Read the model definition and answer for the solid it produces. Units are mm, in the model's axes. Coordinates: 2 decimals unless noted, no trailing zeros. Write each loop counter-clockwise with the first axis right and the second up, starting at its lowest first coordinate (ties: lowest second). Pieces come first, ordered by that corner, then holes. Notation, with made-up numbers: (56, -22) -> (79, -22) arc R19 ccw to (79, -16) -> close; hole circle Ø6 at (-4.75, 5.25). An arc over 180 degrees is marked (long way). Use CSV: the item, a comma, the result in double quotes.
from build123d import *

# Parameters (mm, degrees)
F0_R     = 1.6
F1_DEPTH = 3.175


with BuildPart() as f1:
    # F0 (on Top) → F1 (new body)
    with BuildSketch(Plane.XY):
        with BuildLine():
            Line((-51.6649944294, -13.3350055706), (0, -13.3350055706))
            ThreePointArc((0, -13.3350055706), (13.3350055706, 0), (0, 13.3350055706))
            Line((0, 13.3350055706), (-51.6649944294, 13.3350055706))
            ThreePointArc((-51.6649944294, 13.3350055706), (-55.2005283353, 11.8705394766), (-56.6649944294, 8.3350055706))
            Line((-56.6649944294, 8.3350055706), (-56.6649944294, -8.3350055706))
            ThreePointArc((-56.6649944294, -8.3350055706), (-55.2005283353, -11.8705394766), (-51.6649944294, -13.3350055706))
        make_face()
        with Locations((-46.6649944294, 0)):
            Circle(F0_R, mode=Mode.SUBTRACT)
        with Locations((-36.6649944294, 0)):
            Circle(F0_R, mode=Mode.SUBTRACT)
        with Locations((-26.6649944294, 0)):
            Circle(F0_R, mode=Mode.SUBTRACT)
        with Locations((-16.6649944294, 0)):
            Circle(F0_R, mode=Mode.SUBTRACT)
        Polygon((-2.3131272616, 1.150841372), (-2.4811892868, 1.651717782), (-1.9542535042, 1.6899369317), (-1.992472654, 2.2168727143), (-1.4725868119, 2.1228475389), (-1.3785616365, 2.6427333809), (-0.8983920744, 2.4223718279), (-0.6780305213, 2.90254139), (-0.2677480588, 2.5696895861), (0.0651037451, 2.9799720486), (0.379719552, 2.555544297), (0.8041473037, 2.8701601039), (1.0033279869, 2.380824761), (1.4926633298, 2.5800054442), (1.5638936344, 2.0565092492), (2.0873898293, 2.1277395538), (2.0261940932, 1.6029756981), (2.5509579489, 1.5417799619), (2.3611813253, 1.0487212884), (2.8542399989, 0.8589446648), (2.547806851, 0.4285718633), (2.9781796525, 0.1221387154), (2.574344302, -0.2185063082), (2.9149893256, -0.6223416587), (2.4391262327, -0.8518549247), (2.6686394987, -1.3277180175), (2.1506488918, -1.4316783634), (2.2546092377, -1.9496689703), (1.7270383715, -1.9215441851), (1.6989135863, -2.4491150513), (1.1949116786, -2.2906723188), (1.0364689461, -2.7946742265), (0.5877042905, -2.5158690862), (0.3088991502, -2.9646337418), (-0.0564307197, -2.5829845462), (-0.4380799154, -2.9483144161), (-0.6970199802, -2.4878015876), (-1.1575328087, -2.7467416524), (-1.2938129119, -2.2363009057), (-1.8042536586, -2.3725810089), (-1.80931082, -1.8442852134), (-2.3376066155, -1.8493423749), (-2.2111230752, -1.3363862984), (-2.7240791517, -1.209902758), (-2.4740023355, -0.7445173173), (-2.9393877762, -0.4944405012), (-2.5814309304, -0.105867575), (-2.9700038565, 0.2520892708), (-2.5266587261, 0.5394342163), (-2.8140036716, 0.9827793468), align=None, mode=Mode.SUBTRACT)
    extrude(amount=F1_DEPTH)


solid = f1.part
1. Find the intervals of material crossed by line 1 along Y through (x, z) = (-27, 1.35) (3 decimals); line 2 along X through (y, z) = (2.5, 0.5) (3 decimals); line 3 along Y through (x, z) = (-18, 1.2) (3 decimals), in increasing order.
Solutions:
line 1,"y = -13.335 to -1.565, 1.565 to 13.335"
line 2,"x = -56.665 to -1.404, -1.068 to -0.863, 0.955 to 1.296, 1.504 to 13.099"
line 3,"y = -13.335 to -0.882, 0.882 to 13.335"
2. A cutting plane is placed at B-B (y = -7.5). Give the vertices of the cut face in (x, z) (3 decimals), and give its area (3 significant figures).
Solutions:
outline,"(-56.665, 0) -> (11.026, 0) -> (11.026, 3.175) -> (-56.665, 3.175) -> close"
area,"215 mm^2"
3. A cutting plane is placed at C-C (x = 4). Give the vertices of the cut face in (y, z) (3 decimals).
Solutions:
outline,"(-12.721, 0) -> (12.721, 0) -> (12.721, 3.175) -> (-12.721, 3.175) -> close"
4. For a pull along Y with two mould halves and no side action, classify faces 1 (the flat face through (-25, 13.335, 2)), 2 (the cylindrical face through (-27.844, 1.081, 1.565)), 3 (the flat face through (-22, 0, 0)) as pulls with the +Y half, pulls with the -Y half, needs draft (parallel to the pull), parting line crosses it, or undercut.
Solutions:
face 1,"pulls with the +Y half"
face 2,"undercut"
face 3,"needs draft"
5. Each of these flat-tipped pins is pushed along its axis until it touches: pin 1 Ø2.5 at (x, y) = (-36.66, 0) entering from +Z; pin 2 Ø6 at (x, y) = (-38, -9) entering from -Z; pin 3 Ø1 at (y, z) = (10.5, 2.5) entering from -X; pin 4 Ø1 at (y, z) = (8.5, 0.5) entering from +X. Where does it stop, or does it pass through?
Solutions:
pin 1,"passes through"
pin 2,"stops at z = 0"
pin 3,"stops at x = -56.38"
pin 4,"stops at x = 10.67"
6. A cutting plane is placed at A-A (z = 1.55). Give the number of separate pieces and of enclosed holes in the cut face, and give its area (3 significant figures).
Solutions:
separate pieces,"1"
enclosed holes,"5"
area,"1,720 mm^2"
